Source: CAD feature listing. Evaluate the final solid. Frame: model axes, mm. A direction names the side the tool comes from. Give positions to 0.01 mm unless a question says otherwise; leave off trailing zeros. Loops run counter-clockwise (first coordinate to the right, second up) from the corner with the lowest first, then second, coordinate; pieces in that order, holes last. Notation, with made-up numbers: (81.5, 23.25) -> (95.5, 23.25) arc R23 cw to (95.5, 40.25) -> close; hole circle Ø4 at (-17, 10.5). An arc over 180 degrees is marked (long way). Answer as a JSON object with one key per item and string values. Group by question number.
from build123d import *

# Parameters (mm, degrees)
CYLINDER008_R     = 16
CYLINDER008_DEPTH = 10
CYLINDER007_R     = 14
CYLINDER007_DEPTH = 6.4
CYLINDER006_R     = 14
CYLINDER006_DEPTH = 1
CYLINDER005_R     = 0.4
CYLINDER005_DEPTH = 1
CYLINDER001_R     = 12.6
CYLINDER001_DEPTH = 8
CYLINDER_R        = 15
CYLINDER_DEPTH    = 8
CYLINDER002_R     = 15
CYLINDER002_DEPTH = 1
FILLET_R          = 0.7
FILLET001_R       = 0.7
FILLET002_R       = 0.8
CYLINDER014_R     = 0.4
CYLINDER014_DEPTH = 2
CYLINDER012_R     = 0.41
CYLINDER012_DEPTH = 0.8
CYLINDER013_R     = 0.7
CYLINDER013_DEPTH = 0.55
FILLET003_R       = 0.24
CYLINDER015_R     = 5
CYLINDER015_DEPTH = 0.1


with BuildPart() as cylinder008:
    # Cylinder008 → Cylinder008 (new body)
    with BuildSketch(Plane.XY.offset(4)):
        Circle(CYLINDER008_R)
    extrude(amount=CYLINDER008_DEPTH)


with BuildPart() as cylinder007:
    # Cylinder007 → Cylinder007 (new body)
    with BuildSketch(Plane.XY.offset(1.6)):
        Circle(CYLINDER007_R)
    extrude(amount=CYLINDER007_DEPTH)


with BuildPart() as cylinder006:
    # Cylinder006 → Cylinder006 (new body)
    with BuildSketch(Plane.XY.offset(7)):
        Circle(CYLINDER006_R)
    extrude(amount=CYLINDER006_DEPTH)


with BuildPart() as cylinder005:
    # Cylinder005 → Cylinder005 (new body)
    with BuildSketch(Plane.XY):
        Circle(CYLINDER005_R)
    extrude(amount=CYLINDER005_DEPTH)


with BuildPart() as cylinder001:
    # Cylinder001 → Cylinder001 (new body)
    with BuildSketch(Plane.XY):
        Circle(CYLINDER001_R)
    extrude(amount=CYLINDER001_DEPTH)


with BuildPart() as cut:
    # Cylinder → Cylinder (new body)
    with BuildSketch(Plane.XY):
        Circle(CYLINDER_R)
    extrude(amount=CYLINDER_DEPTH)

    # Cut: cut Cylinder001
    add(cylinder001.part, mode=Mode.SUBTRACT)


with BuildPart() as cut007:
    # Cylinder002 → Cylinder002 (new body)
    with BuildSketch(Plane.XY):
        Circle(CYLINDER002_R)
    extrude(amount=CYLINDER002_DEPTH)

    # Fusion: union Cut
    add(cut.part)

    # Cut001: cut Cylinder005
    add(cylinder005.part, mode=Mode.SUBTRACT)

    # Cut003: cut Cylinder006
    add(cylinder006.part, mode=Mode.SUBTRACT)

    # Fillet
    fillet_edges = [cut007.edges().sort_by_distance(p)[0] for p in [
        (-15, 0, 8),
    ]]
    fillet(fillet_edges, radius=FILLET_R)

    # Fillet001
    fillet001_edges = [cut007.edges().sort_by_distance(p)[0] for p in [
        (-15, 0, 0),
    ]]
    fillet(fillet001_edges, radius=FILLET001_R)

    # Fillet002
    fillet002_edges = [cut007.edges().sort_by_distance(p)[0] for p in [
        (-0.4, 0, 0),
    ]]
    fillet(fillet002_edges, radius=FILLET002_R)

    # Cut004: cut Cylinder007
    add(cylinder007.part, mode=Mode.SUBTRACT)

    # Cut007: cut Cylinder008
    add(cylinder008.part, mode=Mode.SUBTRACT)


with BuildPart() as cylinder014:
    # Cylinder014 → Cylinder014 (new body)
    with BuildSketch(Plane.XY.offset(1)):
        Circle(CYLINDER014_R)
    extrude(amount=CYLINDER014_DEPTH)


with BuildPart() as cylinder012:
    # Cylinder012 → Cylinder012 (new body)
    with BuildSketch(Plane.XY.offset(1)):
        Circle(CYLINDER012_R)
    extrude(amount=CYLINDER012_DEPTH)


with BuildPart() as fillet003:
    # Cylinder013 → Cylinder013 (new body)
    with BuildSketch(Plane.XY.offset(1)):
        Circle(CYLINDER013_R)
    extrude(amount=CYLINDER013_DEPTH)

    # Fusion001: union Cylinder012
    add(cylinder012.part)

    # Fillet003
    fillet003_edges = [fillet003.edges().sort_by_distance(p)[0] for p in [
        (-0.41, 0, 1.55),
    ]]
    fillet(fillet003_edges, radius=FILLET003_R)


with BuildPart() as fusion003:
    # Cylinder015 → Cylinder015 (new body)
    with BuildSketch(Plane.XY.offset(1)):
        Circle(CYLINDER015_R)
    extrude(amount=CYLINDER015_DEPTH)

    # Fusion002: union Fillet003
    add(fillet003.part)

    # Cut006: cut Cylinder014
    add(cylinder014.part, mode=Mode.SUBTRACT)

    # Fusion003: union Cut007
    add(cut007.part)


solid = fusion003.part
(1) Mould query, pull axis Y, two halves, no side actions, for faces 3 (the face through (1, 0, 1.1)), 4 (the face through (-13, 2, 1.6)), 5 (the face through (3, 0, 0)), 6 (the face through (-14.985, 0.66, 2.327)). Classes: pulls with the +Y half, pulls with the -Y half, needs draft (parallel to the pull), parting line crosses it, or undercut.
(2) First-contact query: pin 1 (1.1 mm diameter, centred on x = 0, y = 0, fed in from +Z); pin 2 (8 mm diameter, centred on x = 0.5, y = 9.5, fed in from +Z); pin 3 (1 mm diameter, centred on y = -10.5, z = 1, fed in from +X); pin 4 (8 mm diameter, centred on x = -5, y = -3, fed in from -Z). Flat tips, straight axial feed; report the tip coordinate or a pass-through.
(3) Material intervals for line 1 (X direction, y = 0, z = 1.2); line 2 (X direction, y = 0, z = 3.3), sorted ascending. Write a range as from..to.
(4) Access query for faces 1 (the face through (-0.7, 0, 1.3)), 2 (the face through (-0.32, -0.24, 1.29)). Directions: +Z, -Z, +X, -X, +Y, -Y. A direction counts if a zero-diameter tool reaches every point of the face in a straight line with its end or side. Return the directions, or none.
(5) Section query C-C on z = 2.65. Return the cut outline in (x, y), plus the area to 3 significant figures.
Result:
{
 "1": {"face 3": "undercut", "face 4": "undercut", "face 5": "needs draft", "face 6": "parting line crosses it"},
 "2": {"pin 1": "z = 1.8", "pin 2": "z = 1.6", "pin 3": "x = 11.18", "pin 4": "z = 0"},
 "3": {"line 1": "-15..-12.6, -0.7..-0.4, 0.4..0.7, 12.6..15", "line 2": "-15..-14, 14..15"},
 "4": {"face 1": "+Z", "face 2": "+Z, -Z"},
 "5": {"outline": "circle Ø30 at (0, 0); hole circle Ø28 at (0, 0)", "area": "91.1 mm²"}
}
